Can you work these out from the model? Positions are in its coordinate system, mm. A direction names the side the tool comes from. Give positions to 0.01 mm unless a question says otherwise; leave off trailing zeros. Order: outer loops, then holes, each group sorted by start corner. A loop starts at its lowest first (then second) coordinate and runs counter-clockwise, first axis right, second up. Notation, with made-up numbers: (-21.75, -1.75) -> (-14.75, -1.75) arc R35 cw to (-14.75, 36.25) -> close; hole circle Ø10 at (28.25, -20.75). An arc over 180 degrees is marked (long way). Answer as a JSON object with one key per item and string values.
```python
from build123d import *

# Parameters (mm, degrees)
SKETCH1_R             = 2.6
BOSS_EXTRUDE1_DEPTH   = 1.6
SKETCH2_R             = 3.45
BOSS_EXTRUDE2_DEPTH   = 1.4
M5X0_8_TAPPED_HOLE1_D = 4.2


with BuildPart() as part:
    # Sketch1 → Boss-Extrude1 (new body)
    with BuildSketch(Plane.XY):
        with BuildLine():
            Line((-10, -8.5), (-10, -5))
            Line((-10, -5), (-37.5, -5))
            Line((-37.5, -5), (-40.974341649, -3.841886117))
            ThreePointArc((-40.974341649, -3.841886117), (-41.716863278, -3.295926597), (-42, -2.41886117))
            Line((-42, -2.41886117), (-42, 2.41886117))
            ThreePointArc((-42, 2.41886117), (-41.716863278, 3.295926597), (-40.974341649, 3.841886117))
            Line((-40.974341649, 3.841886117), (-37.5, 5))
            Line((-37.5, 5), (-10, 5))
            Line((-10, 5), (-10, 8.5))
            ThreePointArc((-10, 8.5), (-9.560660172, 9.560660172), (-8.5, 10))
            Line((-8.5, 10), (-5, 10))
            Line((-5, 10), (-5, 37.485))
            Line((-5, 37.485), (-3.841886117, 40.959341649))
            ThreePointArc((-3.841886117, 40.959341649), (-3.295926597, 41.701863278), (-2.41886117, 41.985))
            Line((-2.41886117, 41.985), (2.41886117, 41.985))
            ThreePointArc((2.41886117, 41.985), (3.295926597, 41.701863278), (3.841886117, 40.959341649))
            Line((3.841886117, 40.959341649), (5, 37.485))
            Line((5, 37.485), (5, 10))
            Line((5, 10), (8.5, 10))
            ThreePointArc((8.5, 10), (9.560660172, 9.560660172), (10, 8.5))
            Line((10, 8.5), (10, -8.5))
            ThreePointArc((10, -8.5), (9.560660172, -9.560660172), (8.5, -10))
            Line((8.5, -10), (5, -10))
            Line((5, -10), (5, -37.485))
            Line((5, -37.485), (3.841886117, -40.959341649))
            ThreePointArc((3.841886117, -40.959341649), (3.295926597, -41.701863278), (2.41886117, -41.985))
            Line((2.41886117, -41.985), (-2.41886117, -41.985))
            ThreePointArc((-2.41886117, -41.985), (-3.295926597, -41.701863278), (-3.841886117, -40.959341649))
            Line((-3.841886117, -40.959341649), (-5, -37.485))
            Line((-5, -37.485), (-5, -10))
            Line((-5, -10), (-8.5, -10))
            ThreePointArc((-8.5, -10), (-9.560660172, -9.560660172), (-10, -8.5))
        make_face()
        Circle(SKETCH1_R, mode=Mode.SUBTRACT)
    extrude(amount=BOSS_EXTRUDE1_DEPTH)

    # Sketch2 → Boss-Extrude2 (add)
    with BuildSketch(Plane.XY.offset(1.6)):
        with Locations((0, 14.95)):
            Circle(SKETCH2_R)
        with Locations((0, 34.95)):
            Circle(SKETCH2_R)
        with Locations((0, -14.95)):
            Circle(SKETCH2_R)
        with Locations((0, -34.95)):
            Circle(SKETCH2_R)
        with Locations((-14.95, 0)):
            Circle(SKETCH2_R)
        with Locations((-34.95, 0)):
            Circle(SKETCH2_R)
    extrude(amount=BOSS_EXTRUDE2_DEPTH)

    # M5x0.8 Tapped Hole1 (through all)
    with Locations(Plane.XY.offset(3)):
        with Locations((0, 34.95), (0, 14.95), (0, -14.95), (0, -34.95), (-14.95, 0), (-34.95, 0)):
            Hole(M5X0_8_TAPPED_HOLE1_D / 2)


solid = part.part
```
1. If we section it at A-A on y = -14.95: Please give me the cut outline in (x, z), then the cut area to 3 significant figures.
Worked answers:
{"outline": "(-5, 0) -> (-2.1, 0) -> (-2.1, 3) -> (-3.45, 3) -> (-3.45, 1.6) -> (-5, 1.6) -> close; (2.1, 0) -> (5, 0) -> (5, 1.6) -> (3.45, 1.6) -> (3.45, 3) -> (2.1, 3) -> close", "area": "13.1 mm²"}
2. Will these pins go through, and if not, where does the flat tip stop? pin 1 Ø10 at (x, y) = (-3, 8) entering from -Z; pin 2 Ø0.8 at (x, z) = (-7, 1) entering from +Y; pin 3 Ø7 at (x, y) = (0, 0) entering from +Z; pin 4 Ø0.5 at (y, z) = (17, 0.5) entering from -X.
Worked answers:
{"pin 1": "z = 0", "pin 2": "y = 10", "pin 3": "z = 1.6", "pin 4": "x = -5"}
3. If we section it at D-D on x = -6: Please give me the cut outline in (y, z), then the cut area to 3 significant figures.
Worked answers:
{"outline": "(-10, 0) -> (10, 0) -> (10, 1.6) -> (-10, 1.6) -> close", "area": "32.0 mm²"}
4. For faces 5 (the face through (-2.738, -17.049, 2.29)), 6 (the face through (2.3, 15, 3)), 7 (the face through (10, 0, 1)), 8 (the face through (-10, -7, 1)), 9 (the face through (7, 10, 1)), which set-ups out of +Z, -Z, +X, -X, +Y, -Y let a thin tool reach every point of the face, with its end or its side?
Worked answers:
{"face 5": "+Z", "face 6": "+Z, +X, -X, +Y, -Y", "face 7": "+Z, -Z, +X, +Y, -Y", "face 8": "+Z, -Z, -X, -Y", "face 9": "+Z, -Z, +X, +Y"}
5. If we mould it in two halves opening along X, with no side actions, what happens to faces 1 (the face through (9.57, -9.55, 0.79)), 2 (the face through (0.273, -12.868, 1.479)), 3 (the face through (-5, -24, 1)), 4 (the face through (-7, 10, 1))? For each: +X half, -X half, draft (parallel to the pull), parting line (faces both ways), or undercut.
Worked answers:
{"face 1": "+X half", "face 2": "undercut", "face 3": "-X half", "face 4": "draft"}
6. Please list where these lines run through material, in increasing order: L1, parallel to Y at x = 0, z = 1.4 (3 decimals); L2, parallel to Y at x = -34.95, z = 1.7; L3, parallel to Z at x = 1, y = -21.5.
Worked answers:
{"L1": "-41.985 to -37.05, -32.85 to -17.05, -12.85 to -2.6, 2.6 to 12.85, 17.05 to 32.85, 37.05 to 41.985", "L2": "-3.45 to -2.1, 2.1 to 3.45", "L3": "0 to 1.6"}
7. If we section it at C-C on x = 0: Count the separate pieces of the cut face and the enclosed holes in it, then the cut area to 3 significant figures.
Worked answers:
{"separate pieces": "6", "enclosed holes": "0", "area": "114 mm²"}
